The listing builds one solid part. Answer for the finished solid, in the listing's coordinates (mm). A direction names the side the tool comes from. Coordinates: 2 decimals unless noted, no trailing zeros. Order: outer loops, then holes, each group sorted by start corner. A loop starts at its lowest first (then second) coordinate and runs counter-clockwise, first axis right, second up. Notation, with made-up numbers: (17, 10.5) -> (67, 10.5) arc R16 ccw to (67, 29.5) -> close; hole circle Ø5 at (17, 6). An arc over 180 degrees is marked (long way). Return JSON: item names as keys, results as strings.
```python
from build123d import *

# Parameters (mm, degrees)
F0_W      = 24
F0_H      = 127
F1_DEPTH  = 33.5
F2_W      = 6
F2_H      = 127
F3_DEPTH  = 19.9
F5_W      = 24
F5_H      = 127
F6_DEPTH  = 10
F7_W      = 85.2
F7_H      = 33.5
F7_H_2    = 10
F8_DEPTH  = 15
F4_R      = 2.25
F9_DEPTH  = 33.5
F11_ANGLE = 90
F12_W     = 63.4
F12_H     = 127
F13_DEPTH = 4
F14_W     = 80.3440480709
F14_H     = 136.8158757687
F15_DEPTH = 1.5
F16_R     = 5


with BuildPart() as f1:
    # F0 (on Top) → F1 (new body)
    with BuildSketch(Plane.XY):
        Rectangle(F0_W, F0_H)
    extrude(amount=F1_DEPTH)

    # F2 (on face) → F3 (join)
    with BuildSketch(Plane.XY.offset(33.5)):
        with Locations((9, 0)):
            Rectangle(F2_W, F2_H)
    extrude(amount=F3_DEPTH)

    # F5 (on face) → F6 (join)
    with BuildSketch(Plane.XY.offset(53.4)):
        Rectangle(F5_W, F5_H)
    extrude(amount=F6_DEPTH)

    # F7 (on face) → F8 (cut)
    with BuildSketch(Plane(origin=(-12, 0, 0), x_dir=(0, -1, 0), z_dir=(-1, 0, 0))):
        with Locations((0, 16.75)):
            Rectangle(F7_W, F7_H)
        with Locations((0, 58.4)):
            Rectangle(F7_W, F7_H_2)
    extrude(amount=-F8_DEPTH, mode=Mode.SUBTRACT)

    # F4 (on face) → F9 (cut, through all)
    with BuildSketch(Plane.XY.offset(33.5)):
        with Locations((0, 53.05)):
            Circle(F4_R)
        with Locations((0, -53.05)):
            Circle(F4_R)
    extrude(amount=-F9_DEPTH, mode=Mode.SUBTRACT)


with BuildPart() as f1_1:
    # F11: moved
    add(f1.part.rotate(Axis((0, -2.2393353283, 0), (0, 1, 0)), F11_ANGLE))

    # F12 (on face) → F13 (cut)
    with BuildSketch(Plane.XY.offset(12)):
        with Locations((31.7, 0)):
            Rectangle(F12_W, F12_H)
    extrude(amount=-F13_DEPTH, mode=Mode.SUBTRACT)

    # F14 (on face) → F15 (join)
    with BuildSketch(Plane(origin=(0, 0, -12), x_dir=(1, 0, 0), z_dir=(0, 0, -1))):
        with Locations((31.7, 0)):
            Rectangle(F14_W, F14_H)
    extrude(amount=-F15_DEPTH)

    # F16
    f16_edges = [f1_1.edges().sort_by_distance(p)[0] for p in [
        (63.4, 63.5, -1.25),
        (0, 63.5, -1.25),
        (-8.472024, 68.407938, -11.25),
        (71.872024, 68.407938, -11.25),
        (0, -63.5, -1.25),
        (63.4, -63.5, -1.25),
        (71.872024, -68.407938, -11.25),
        (-8.472024, -68.407938, -11.25),
    ]]
    fillet(f16_edges, radius=F16_R)


solid = f1_1.part
```
Item 1: Determine the mould class of faces 5 (the flat face through (17, 42.6, 3)), 6 (the cylindrical face through (1.5, -62.07, -1.38)), 7 (the flat face through (58, -42.6, 3)), 8 (the flat face through (0, 1, -5)) for opening direction Y: pulls with the +Y half, pulls with the -Y half, needs draft (parallel to the pull), parting line crosses it, or undercut.
Answer list:
{"face 5": "undercut", "face 6": "pulls with the -Y half", "face 7": "undercut", "face 8": "needs draft"}
Item 2: The part is cut by section D-D on x = 42.5. Determine the outline of the cut face in (y, z).
Answer list:
{"outline": "(-68.41, -12) -> (68.41, -12) -> (68.41, -10.5) -> (63.5, -10.5) -> (63.5, -6) -> (-63.5, -6) -> (-63.5, -10.5) -> (-68.41, -10.5) -> close"}
Item 3: The part is cut by section B-B on z = 0. Determine the outline of the cut face in (x, y), plus the area to 3 significant figures.
Answer list:
{"outline": "(0, -58.5) arc R5 ccw to (5, -63.5) -> (33.5, -63.5) -> (33.5, -55.3) -> (0, -55.3) -> close; (0, -50.8) -> (33.5, -50.8) -> (33.5, -42.6) -> (0, -42.6) -> close; (0, 42.6) -> (33.5, 42.6) -> (33.5, 50.8) -> (0, 50.8) -> close; (0, 55.3) -> (33.5, 55.3) -> (33.5, 63.5) -> (5, 63.5) arc R5 ccw to (0, 58.5) -> close; (53.4, -63.5) -> (58.4, -63.5) arc R5 ccw to (63.4, -58.5) -> (63.4, -42.6) -> (53.4, -42.6) -> close; (53.4, 42.6) -> (63.4, 42.6) -> (63.4, 58.5) arc R5 ccw to (58.4, 63.5) -> (53.4, 63.5) -> close", "area": "1,500 mm2"}
Item 4: The part is cut by section C-C on y = 37.5. Determine the outline of the cut face in (x, z).
Answer list:
{"outline": "(-8.47, -12) -> (71.87, -12) -> (71.87, -10.5) -> (63.4, -10.5) -> (63.4, -3) -> (53.4, -3) -> (53.4, -6) -> (33.5, -6) -> (33.5, -3) -> (0, -3) -> (0, -10.5) -> (-8.47, -10.5) -> close"}
Item 5: The part is cut by section A-A on y = -53.05. Determine the outline of the cut face in (x, z), plus the area to 3 significant figures.
Answer list:
{"outline": "(-8.47, -12) -> (71.87, -12) -> (71.87, -10.5) -> (63.4, -10.5) -> (63.4, 8) -> (53.4, 8) -> (53.4, -6) -> (33.5, -6) -> (33.5, -2.25) -> (0, -2.25) -> (0, -10.5) -> (-8.47, -10.5) -> close; (0, 2.25) -> (33.5, 2.25) -> (33.5, 8) -> (0, 8) -> close", "area": "864 mm2"}
Item 6: Which of the six approach directions +Z, -Z, +X, -X, +Y, -Y give full straight-line access (tool end or side, diameter ignored) to faces 1 (the cylindrical face through (16.984, 51.054, -1.038)), 2 (the cylindrical face through (61.97, -62, -1.38)), 3 (the flat face through (33.5, 15, -4)), 4 (the cylindrical face through (61.97, 62, -1.38))?
Answer list:
{"face 1": "-X", "face 2": "+Z, +X, -Y", "face 3": "+Z, +Y, -Y", "face 4": "+Z, +X, +Y"}
Item 7: Flat-ended cylindrical pins translate along their axes: pin 1 (8 mm diameter, centred on x = 58.5, z = 4, fed in from +Y); pin 2 (10 mm diameter, centred on y = -1.5, z = 5, fed in from +X); pin 3 (5 mm diameter, centred on x = 60.5, y = 1.5, fed in from +Z); pin 4 (1.5 mm diameter, centred on y = 54, z = 6, fed in from -X). Find the tip coordinate at first contact, or state that the pin passes through.
Answer list:
{"pin 1": "y = 63.5", "pin 2": "through", "pin 3": "z = -3", "pin 4": "x = 0"}
Item 8: Find the intervals of material crossed by probe 1 along Y at (x, z) = (8, 0); probe 2 along X at (y, z) = (-57.5, 7); probe 3 along Z at (x, y) = (12, -53), in increasing order.
Answer list:
{"probe 1": "-63.5 to -55.3, -50.8 to -42.6, 42.6 to 50.8, 55.3 to 63.5", "probe 2": "0 to 33.5, 53.4 to 63.4", "probe 3": "-12 to -2.25, 2.25 to 8"}
